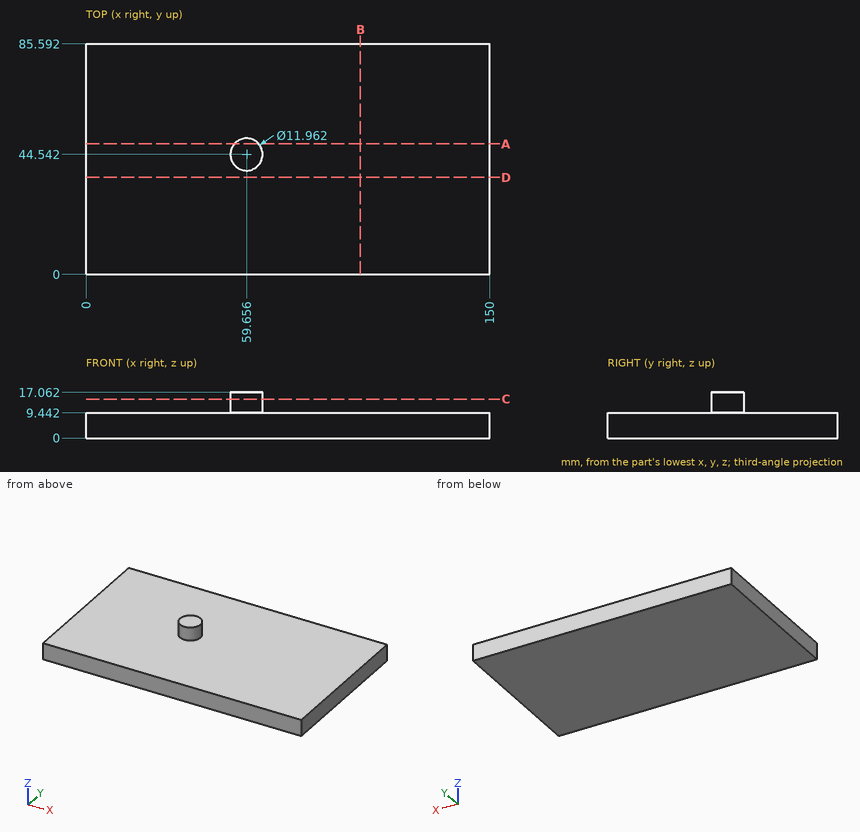
Input: dimensioned drawing with shaded views. Units: mm. Origin: part minimum x, y, z. Round coordinates to 2 decimals unless told otherwise and drop trailing zeros. Loops run counter-clockwise (first coordinate to the right, second up) from the corner with the lowest first, then second, coordinate; pieces in that order, holes last.
1) Section query B-B on x = 102. Return the cut outline in (y, z), plus the area to 3 significant figures.
Ans:
outline: (0, 0) - (85.59, 0) - (85.59, 9.44) - (0, 9.44) - close
area: 808 mm2
2) Section query A-A on y = 48.5. Return the cut outline in (x, z).
Ans:
outline: (0, 0) - (150, 0) - (150, 9.44) - (64.14, 9.44) - (64.14, 17.06) - (55.17, 17.06) - (55.17, 9.44) - (0, 9.44) - close
3) Material intervals for line 1 (Z direction, x = 81, y = 33); line 2 (X direction, y = 44, z = 10.5); line 3 (X direction, y = 43, z = 10) (1 decimal), sorted ascending.
Ans:
line 1: z = 0 to 9.44
line 2: x = 53.7 to 65.61
line 3: x = 53.9 to 65.4
4) Section query C-C on z = 14.5. Return the cut outline in (x, y) (1 decimal).
Ans:
outline: circle Ø12 at (59.7, 44.5)
5) Section query D-D on y = 36. Return the cut outline in (x, z).
Ans:
outline: (0, 0) - (150, 0) - (150, 9.44) - (0, 9.44) - close
